Source: CAD feature listing. Evaluate the final solid. Frame: model axes, mm. A direction names the side the tool comes from. Coordinates: 2 decimals unless noted, no trailing zeros. Loops run counter-clockwise (first coordinate to the right, second up) from the corner with the lowest first, then second, coordinate; pieces in that order, holes last.
from build123d import *

# Parameters (mm, degrees)
F1_R      = 7.5
F3_R      = 12.5
F4_DEPTH  = 12.5
F5_R      = 6
F6_DEPTH  = 25
F9_DEPTH  = 12.5
F10_R     = 6
F11_DEPTH = 25


with BuildPart() as f2:
    # F2: sweep along a path in F0
    with BuildLine(Plane.XY) as f2_path:
        Line((150, -12), (125, -12))
        ThreePointArc((125, -12), (81.789999989, -9.4166667579), (39.1955835962, -1.7034700315))
        ThreePointArc((39.1955835962, -1.7034700315), (32.1487132371, -0.4273896908), (25, 0))
        Line((25, 0), (0, 0))
    # F1 (on Right) → F2 (sweep)
    with BuildSketch(Plane.YZ):
        Circle(F1_R)
    sweep(path=f2_path.line)

    # F3 (on Front) → F4 (join, symmetric)
    with BuildSketch(Plane.XZ):
        Circle(F3_R)
    extrude(amount=F4_DEPTH, both=True)

    # F5 (on face) → F6 (cut)
    with BuildSketch(Plane.XZ.offset(12.5)):
        Circle(F5_R)
    extrude(amount=-F6_DEPTH, mode=Mode.SUBTRACT)

    # F8 (on offset) → F9 (join, symmetric)
    with BuildSketch(Plane.XZ.offset(12)):
        with BuildLine():
            Line((150, 7.5), (150, -7.5))
            Line((150, -7.5), (140, -7.5))
            ThreePointArc((140, -7.5), (153.9528470752, -11.8585412256), (162.5, 0))
            ThreePointArc((162.5, 0), (153.9528470752, 11.8585412256), (140, 7.5))
            Line((140, 7.5), (150, 7.5))
        make_face()
        with BuildLine():
            Line((140, -7.5), (150, -7.5))
            Line((150, -7.5), (150, 7.5))
            Line((150, 7.5), (140, 7.5))
            ThreePointArc((140, 7.5), (137.5, 0), (140, -7.5))
        make_face()
    extrude(amount=F9_DEPTH, both=True)

    # F10 (on face) → F11 (cut)
    with BuildSketch(Plane.XZ.offset(24.5)):
        with Locations((150, 0)):
            Circle(F10_R)
    extrude(amount=-F11_DEPTH, mode=Mode.SUBTRACT)


solid = f2.part
Q1. Section A-A, the plane x = 0. Return the cut outline in (y, z).
Q2. Line query: line 1 along Z through (x, y) = (0, -1); line 2 along X through (y, z) = (9, -5.25); line 3 along X through (y, z) = (8.5, -3.25). Output: solid intervals per line, ascending.
Q3. Access query for faces 1 (the flat face through (-3, 12.5, -5.4)), 2 (the flat face through (147, 0.5, -5.4)), 3 (the cylindrical face through (17.4, 6.93, 2.87)). Directions: +Z, -Z, +X, -X, +Y, -Y. A direction counts if a zero-diameter tool reaches every point of the face in a straight line with its end or side. Return the directions, or none.
Q4. Section C-C, the plane z = 9. Return the cut outline in (x, y).
Q5. Section B-B, the plane z = -3. Return the cut outline in (x, y), plus the area to 3 significant figures.
Q6. Section D-D, the plane y = 9. Return the cut outline in (x, z), plus the area to 3 significant figures.
Q7. Contact query for flat-ended pins moving along their axis: pin 1 Ø12 at (y, z) = (8, -7) entering from -X; pin 2 Ø1 at (y, z) = (8.5, 4.5) entering from +X; pin 3 Ø1 at (y, z) = (-1, 7.5) entering from -X. Output: stop coordinate, or through.
Q8. Draft query along X for faces 4 (the cylindrical face through (145.24, -12.18, -3.65)), 5 (the flat face through (-3, -12.5, -5.4)). Return one class per face: +X half, -X half, draft (parallel to the pull), parting line (faces both ways), or undercut.
Derived:
1. outline: (-12.5, -12.5) - (12.5, -12.5) - (12.5, -6) - (-12.5, -6) - close; (-12.5, 6) - (12.5, 6) - (12.5, 12.5) - (-12.5, 12.5) - close
2. line 1: z = -12.5 to -6, 6 to 12.5
2. line 2: x = -11.34 to -2.9, 2.9 to 11.34
2. line 3: x = -12.07 to -5.04, 5.04 to 12.07
3. face 1: +Z, -Z, +X, -X, +Y
3. face 2: +Z, -Z, +X, +Y
3. face 3: none
4. outline: (-8.67, -12.5) - (8.67, -12.5) - (8.67, 12.5) - (-8.67, 12.5) - close; (141.33, -24.5) - (158.67, -24.5) - (158.67, 0.5) - (141.33, 0.5) - close
5. outline: (-12.13, -12.5) - (-5.2, -12.5) - (-5.2, 12.5) - (-12.13, 12.5) - close; (5.2, -12.5) - (12.13, -12.5) - (12.13, -6.87) - (25, -6.87) arc R53.13 cw to (37.57, -8.38) arc R369.54 ccw to (125, -18.87) - (137.87, -18.87) - (137.87, -24.5) - (144.8, -24.5) - (144.8, 0.5) - (137.87, 0.5) - (137.87, -5.13) - (125, -5.13) arc R355.79 cw to (40.82, 4.98) arc R66.87 ccw to (25, 6.87) - (12.13, 6.87) - (12.13, 12.5) - (5.2, 12.5) - close; (155.2, -24.5) - (162.13, -24.5) - (162.13, 0.5) - (155.2, 0.5) - close
5. area: 2,440 mm2
6. outline: circle Ø25 at (0, 0); hole circle Ø12 at (0, 0)
6. area: 378 mm2
7. pin 1: stops at x = -12.46
7. pin 2: stops at x = 11.84
7. pin 3: stops at x = -10.36
8. face 4: undercut
8. face 5: draft
